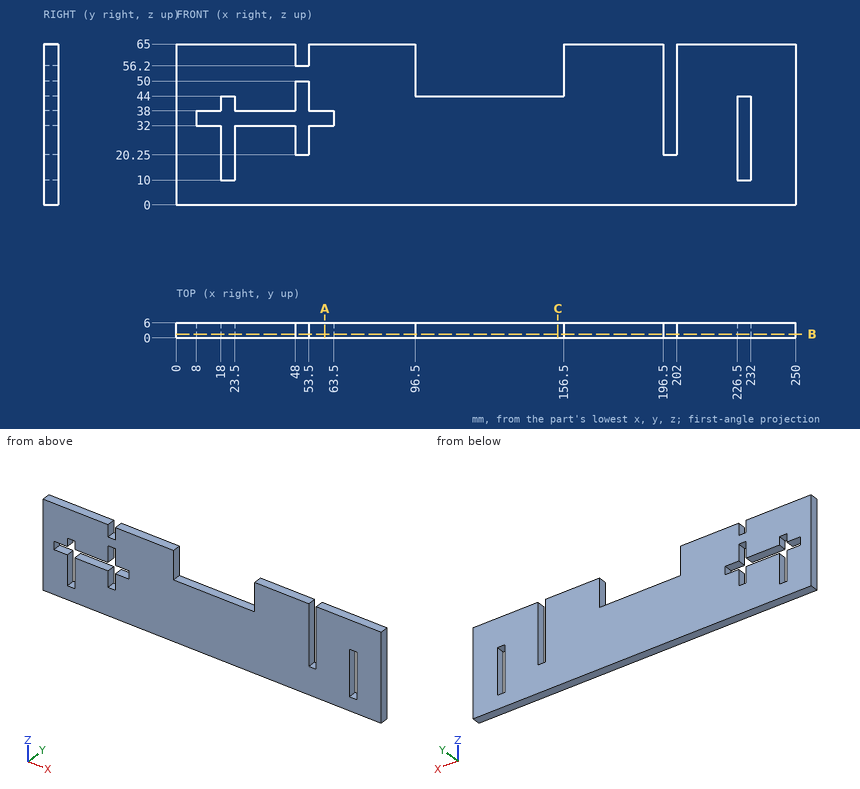
Part print with two shaded views. Sizes in mm from the minimum x, y, z corner. Give positions to 0.01 mm unless a question says otherwise; leave off trailing zeros. Loops run counter-clockwise (first coordinate to the right, second up) from the corner with the lowest first, then second, coordinate; pieces in that order, holes last. Notation, with made-up numbers: (-15.5, 29.25) - (-10.5, 29.25) arc R29 ccw to (-10.5, 63.25) - close; hole circle Ø10 at (72, 56.5). An arc over 180 degrees is marked (long way). Put each result on its own line as item: value.
Q1. Probe line 1 along X through (y, z) = (0.35, 40.5); line 2 along X through (y, z) = (4.8, 59.5); line 3 along Z through (x, y) = (51, 2.2). List the from-to ranges inside material, lowest first.
Filled in:
line 1: x = 0 to 18, 23.5 to 48, 53.5 to 196.5, 202 to 226.5, 232 to 250
line 2: x = 0 to 48, 53.5 to 96.5, 156.5 to 196.5, 202 to 250
line 3: z = 0 to 20.25, 50 to 56.2
Q2. Slice it at A-A (x = 60). Give the cut face in (y, z), plus the area to 3 significant figures.
Filled in:
outline: (0, 0) - (6, 0) - (6, 32) - (0, 32) - close; (0, 38) - (6, 38) - (6, 65) - (0, 65) - close
area: 354 mm²
Q3. Slice it at B-B (y = 1.5). Give the number of separate pieces and of enclosed holes in the cut face, plus the area to 3 significant figures.
Filled in:
separate pieces: 1
enclosed holes: 2
area: 13,900 mm²
Q4. Slice it at C-C (x = 154). Give the cut face in (y, z).
Filled in:
outline: (0, 0) - (6, 0) - (6, 44) - (0, 44) - close
